The drawing under review shows one solid part. Ordinate dimensions are in mm from its lowest x, y, z. Give positions to 0.01 mm unless a question says otherwise; leave off trailing zeros. Write each loop counter-clockwise with the first axis right and the second up, starting at its lowest first coordinate (ties: lowest second). Pieces come first, ordered by that corner, then holes. Notation, with made-up numbers: (49.5, -10) -> (59.5, -10) arc R26 cw to (59.5, 21) -> close; hole circle Ø8 at (60.25, -22.75). An arc over 180 degrees is marked (long way). Answer as a JSON object with one key per item and string values.
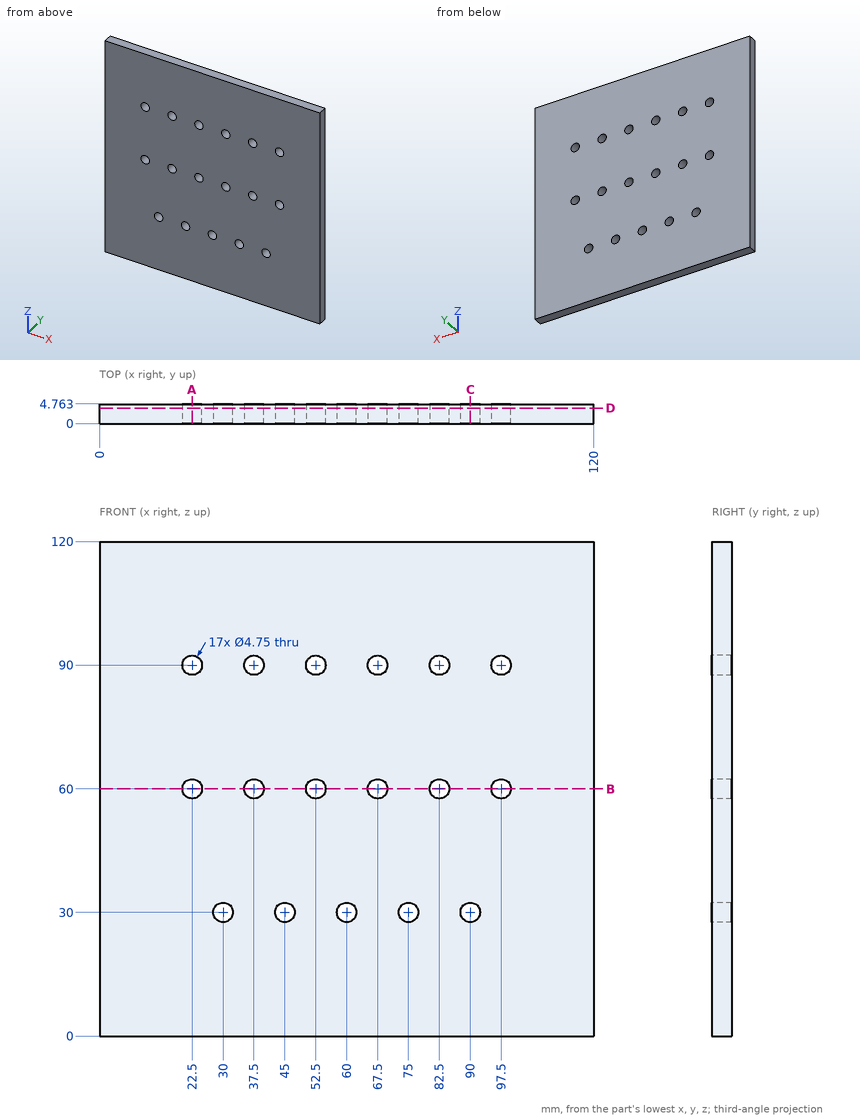
(1) We need section B-B, the plane z = 60. State the section outline as (x, y) points (1 decimal).
Here are the results:
{"outline": "(0, 0) -> (20.1, 0) -> (20.1, 4.8) -> (0, 4.8) -> close; (24.9, 0) -> (35.1, 0) -> (35.1, 4.8) -> (24.9, 4.8) -> close; (39.9, 0) -> (50.1, 0) -> (50.1, 4.8) -> (39.9, 4.8) -> close; (54.9, 0) -> (65.1, 0) -> (65.1, 4.8) -> (54.9, 4.8) -> close; (69.9, 0) -> (80.1, 0) -> (80.1, 4.8) -> (69.9, 4.8) -> close; (84.9, 0) -> (95.1, 0) -> (95.1, 4.8) -> (84.9, 4.8) -> close; (99.9, 0) -> (120, 0) -> (120, 4.8) -> (99.9, 4.8) -> close"}
(2) We need section D-D, the plane y = 3.75. Give the number of separate pieces and of enclosed holes in the cut face, then the cut area to 3 significant figures.
Here are the results:
{"separate pieces": "1", "enclosed holes": "17", "area": "14,100 mm²"}
(3) For line 1 along Z through (x, y) = (82.5, 2.35) (1 decimal); line 2 along X through (y, z) = (3.7, 30) (1 decimal); line 3 along Z through (x, y) = (90, 1.6) (1 decimal), list the stretches that pass through material, from the lowest coordinate up.
Here are the results:
{"line 1": "z = 0 to 57.6, 62.4 to 87.6, 92.4 to 120", "line 2": "x = 0 to 27.6, 32.4 to 42.6, 47.4 to 57.6, 62.4 to 72.6, 77.4 to 87.6, 92.4 to 120", "line 3": "z = 0 to 27.6, 32.4 to 120"}
(4) We need section A-A, the plane x = 22.5. State the section outline as (y, z) points (1 decimal).
Here are the results:
{"outline": "(0, 0) -> (4.8, 0) -> (4.8, 57.6) -> (0, 57.6) -> close; (0, 62.4) -> (4.8, 62.4) -> (4.8, 87.6) -> (0, 87.6) -> close; (0, 92.4) -> (4.8, 92.4) -> (4.8, 120) -> (0, 120) -> close"}
(5) We need section C-C, the plane x = 90. State the section outline as (y, z) points (1 decimal), then the cut area to 3 significant figures.
Here are the results:
{"outline": "(0, 0) -> (4.8, 0) -> (4.8, 27.6) -> (0, 27.6) -> close; (0, 32.4) -> (4.8, 32.4) -> (4.8, 120) -> (0, 120) -> close", "area": "549 mm²"}
